Here's how the part is built. I have some questions about the finished solid (model axes, mm). Face numbers are marked on the shaded views. A direction names the side the tool comes from. Round coordinates to 2 decimals unless told otherwise and drop trailing zeros. Order: outer loops, then holes, each group sorted by start corner. A loop starts at its lowest first (then second) coordinate and runs counter-clockwise, first axis right, second up. Notation, with made-up numbers: (70, -39.75) -> (123, -39.75) arc R5 cw to (123, -31.75) -> close; hole circle Ø11 at (-14.75, 82). An arc over 180 degrees is marked (long way). Answer in a Markdown table with one row per item.
```python
from build123d import *

# Parameters (mm, degrees)
SKETCH_2_W          = 140
SKETCH_2_H          = 140
EXTRUDE_1_DEPTH     = 4
EXTRUDE_1_2_DEPTH   = 100
EXTRUDE_2_DEPTH     = 2
CUT_EXTRUDE_1_DEPTH = 105.5
SKETCH_6_R          = 6.5
CUT_EXTRUDE_2_DEPTH = 5
FILLET_1_R          = 10
CUT_EXTRUDE_3_REACH = 106


with BuildPart() as part:
    # Эскиз2 → Extrude 1 (new body)
    with BuildSketch(Plane(origin=(0, 0, 0), x_dir=(1, 0, 0), z_dir=(0, 1, 0))):
        Rectangle(SKETCH_2_W, SKETCH_2_H)
    extrude(amount=EXTRUDE_1_DEPTH)

    # Эскиз3 → Extrude 1 2 (add)
    with BuildSketch(Plane(origin=(0, 4, 0), x_dir=(1, 0, 0), z_dir=(0, 1, 0))):
        with BuildLine():
            Line((-30.5, -30), (-30.5, 29))
            ThreePointArc((-30.5, 29), (-30.207106781, 29.707106781), (-29.5, 30))
            Line((-29.5, 30), (29.5, 30))
            ThreePointArc((29.5, 30), (30.207106781, 29.707106781), (30.5, 29))
            Line((30.5, 29), (30.5, -30))
            Line((30.5, -30), (34.5, -30))
            Line((34.5, -30), (34.5, 29))
            ThreePointArc((34.5, 29), (33.035533906, 32.535533906), (29.5, 34))
            Line((29.5, 34), (-29.5, 34))
            ThreePointArc((-29.5, 34), (-33.035533906, 32.535533906), (-34.5, 29))
            Line((-34.5, 29), (-34.5, -30))
            Line((-34.5, -30), (-30.5, -30))
        make_face()
    extrude(amount=EXTRUDE_1_2_DEPTH)

    # Эскиз4 → Бобышка-Вытянуть2 (add, symmetric)
    with BuildSketch(Plane(origin=(0, 0, 0), x_dir=(0, 0, -1), z_dir=(1, 0, 0))):
        Polygon((34, 57.693575035), (65, 4), (34, 4), align=None)
    extrude(amount=EXTRUDE_2_DEPTH, both=True)

    # Эскиз5 → Вырез-Вытянуть1 (cut, through all)
    with BuildSketch(Plane(origin=(34.5, 0, 0), x_dir=(0, 0, -1), z_dir=(1, 0, 0))):
        with BuildLine():
            Line((-10, 92), (-10, 80))
            ThreePointArc((-10, 80), (-15, 75), (-20, 80))
            Line((-20, 80), (-20, 92))
            ThreePointArc((-20, 92), (-15, 97), (-10, 92))
        make_face()
        with BuildLine():
            Line((-10, 28), (-10, 16))
            ThreePointArc((-10, 16), (-15, 11), (-20, 16))
            Line((-20, 16), (-20, 28))
            ThreePointArc((-20, 28), (-15, 33), (-10, 28))
        make_face()
        with BuildLine():
            Line((10, 92), (10, 80))
            ThreePointArc((10, 80), (15, 75), (20, 80))
            Line((20, 80), (20, 92))
            ThreePointArc((20, 92), (15, 97), (10, 92))
        make_face()
        with BuildLine():
            Line((10, 28), (10, 16))
            ThreePointArc((10, 16), (15, 11), (20, 16))
            Line((20, 16), (20, 28))
            ThreePointArc((20, 28), (15, 33), (10, 28))
        make_face()
    extrude(amount=-CUT_EXTRUDE_1_DEPTH, mode=Mode.SUBTRACT)

    # Эскиз6 → Вырез-Вытянуть2 (cut, through all)
    with BuildSketch(Plane(origin=(0, 4, 0), x_dir=(1, 0, 0), z_dir=(0, 1, 0))):
        with Locations(Location((-55, 55, 0), (0, 0, 270))):  # turned: the seam where the file's is
            Circle(SKETCH_6_R)
        with Locations(Location((-55, -55, 0), (0, 0, 270))):  # turned: the seam where the file's is
            Circle(SKETCH_6_R)
        with Locations(Location((55, 55, 0), (0, 0, 270))):  # turned: the seam where the file's is
            Circle(SKETCH_6_R)
        with Locations(Location((55, -55, 0), (0, 0, 270))):  # turned: the seam where the file's is
            Circle(SKETCH_6_R)
    extrude(amount=-CUT_EXTRUDE_2_DEPTH, mode=Mode.SUBTRACT)

    # Скругление1
    fillet_1_edges = [part.edges().sort_by_distance(p)[0] for p in [
        (70, 2, 70),
        (-70, 2, 70),
        (-70, 2, -70),
        (70, 2, -70),
    ]]
    fillet(fillet_1_edges, radius=FILLET_1_R)

    # Эскиз8 → Вырез-Вытянуть3 (cut, up to next)
    with BuildSketch(Plane(origin=(0, 0, -34), x_dir=(-1, 0, 0), z_dir=(0, 0, -1)), mode=Mode.PRIVATE) as cut_extrude_3_sk1:
        with BuildLine():
            Line((-10, 92), (-10, 80))
            ThreePointArc((-10, 80), (-15, 75), (-20, 80))
            Line((-20, 80), (-20, 92))
            ThreePointArc((-20, 92), (-15, 97), (-10, 92))
        make_face()
    cut_extrude_3_tool1 = extrude(cut_extrude_3_sk1.sketch, amount=-CUT_EXTRUDE_3_REACH, mode=Mode.PRIVATE) & part.part
    add(cut_extrude_3_tool1.solids().sort_by_distance((15, 86, -34))[0], mode=Mode.SUBTRACT)
    # Эскиз8 → Вырез-Вытянуть3 (cut, up to next)
    with BuildSketch(Plane(origin=(0, 0, -34), x_dir=(-1, 0, 0), z_dir=(0, 0, -1)), mode=Mode.PRIVATE) as cut_extrude_3_sk2:
        with BuildLine():
            Line((-10, 28), (-10, 16))
            ThreePointArc((-10, 16), (-15, 11), (-20, 16))
            Line((-20, 16), (-20, 28))
            ThreePointArc((-20, 28), (-15, 33), (-10, 28))
        make_face()
    cut_extrude_3_tool2 = extrude(cut_extrude_3_sk2.sketch, amount=-CUT_EXTRUDE_3_REACH, mode=Mode.PRIVATE) & part.part
    add(cut_extrude_3_tool2.solids().sort_by_distance((15, 22, -34))[0], mode=Mode.SUBTRACT)
    # Эскиз8 → Вырез-Вытянуть3 (cut, up to next)
    with BuildSketch(Plane(origin=(0, 0, -34), x_dir=(-1, 0, 0), z_dir=(0, 0, -1)), mode=Mode.PRIVATE) as cut_extrude_3_sk3:
        with BuildLine():
            Line((10, 92), (10, 80))
            ThreePointArc((10, 80), (15, 75), (20, 80))
            Line((20, 80), (20, 92))
            ThreePointArc((20, 92), (15, 97), (10, 92))
        make_face()
    cut_extrude_3_tool3 = extrude(cut_extrude_3_sk3.sketch, amount=-CUT_EXTRUDE_3_REACH, mode=Mode.PRIVATE) & part.part
    add(cut_extrude_3_tool3.solids().sort_by_distance((-15, 86, -34))[0], mode=Mode.SUBTRACT)
    # Эскиз8 → Вырез-Вытянуть3 (cut, up to next)
    with BuildSketch(Plane(origin=(0, 0, -34), x_dir=(-1, 0, 0), z_dir=(0, 0, -1)), mode=Mode.PRIVATE) as cut_extrude_3_sk4:
        with BuildLine():
            Line((10, 28), (10, 16))
            ThreePointArc((10, 16), (15, 11), (20, 16))
            Line((20, 16), (20, 28))
            ThreePointArc((20, 28), (15, 33), (10, 28))
        make_face()
    cut_extrude_3_tool4 = extrude(cut_extrude_3_sk4.sketch, amount=-CUT_EXTRUDE_3_REACH, mode=Mode.PRIVATE) & part.part
    add(cut_extrude_3_tool4.solids().sort_by_distance((-15, 22, -34))[0], mode=Mode.SUBTRACT)


solid = part.part
```
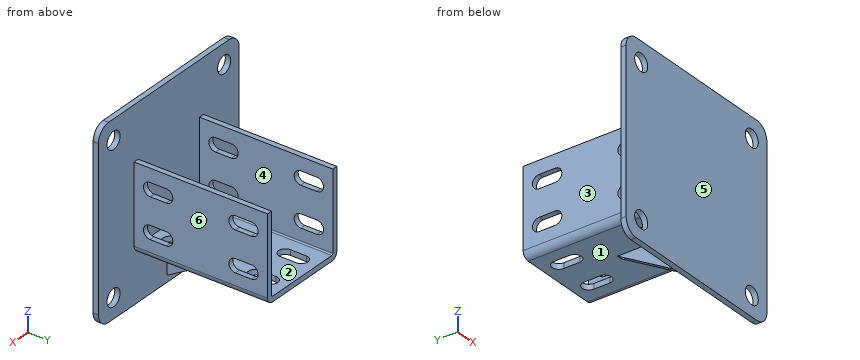
1. For the marked faces 1 and 2, which set-ups out of +Z, -Z, +X, -X, +Y, -Y let a thin tool reach every point of the face, with its end or its side?
Numbers:
| item | result |
|---|---|
| face 1 | -Z, +Y |
| face 2 | +Z, +Y |
2. For pin 1 Ø1.2 at (x, y) = (33, 88) entering from -Z; pin 2 Ø2 at (y, z) = (22, -32) entering from -X; pin 3 Ø3 at (x, z) = (-39, 53) entering from +Y, each with a flat end and sliding along its axis, tell me the tip position at first contact or that it passes through.
Numbers:
| item | result |
|---|---|
| pin 1 | stops at z = -33.07 |
| pin 2 | stops at x = -34.08 |
| pin 3 | stops at y = 4 |
3. We'd pull the mould along X, two halves only. Please class the marked faces 3, 4, 5 and 6: released by +X, released by -X, zero draft, split by the parting line, or undercut.
Numbers:
| item | result |
|---|---|
| face 3 | released by -X |
| face 4 | undercut |
| face 5 | zero draft |
| face 6 | released by +X |
4. Suppose I cut it at D-D on x = 15. Write out the boundary of the cut face in (y, z), then the cut area to 3 significant figures.
Numbers:
| item | result |
|---|---|
| outline | (0, -70) -> (4, -70) -> (4, -34) -> (11, -34) -> (11, -30) -> (4, -30) -> (4, 70) -> (0, 70) -> close; (33, -34) -> (75, -34) -> (75, -30) -> (33, -30) -> close; (97, -34) -> (104, -34) -> (104, -30) -> (97, -30) -> close |
| area | 784 mm2 |
5. Suppose I cut it at B-B on z = -15. Write out the boundary of the cut face in (x, y).
Numbers:
| item | result |
|---|---|
| outline | (-70, 0) -> (70, 0) -> (70, 4) -> (34.5, 4) -> (34.5, 11) -> (30.5, 11) -> (30.5, 4) -> (-30.5, 4) -> (-30.5, 11) -> (-34.5, 11) -> (-34.5, 4) -> (-70, 4) -> close; (-34.5, 33) -> (-30.5, 33) -> (-30.5, 75) -> (-34.5, 75) -> close; (-34.5, 97) -> (-30.5, 97) -> (-30.5, 104) -> (-34.5, 104) -> close; (30.5, 33) -> (34.5, 33) -> (34.5, 75) -> (30.5, 75) -> close; (30.5, 97) -> (34.5, 97) -> (34.5, 104) -> (30.5, 104) -> close |
6. Suppose I cut it at C-C on y = 61. Write out the boundary of the cut face in (x, z).
Numbers:
| item | result |
|---|---|
| outline | (-34.5, -29) arc R5 ccw to (-29.5, -34) -> (29.5, -34) arc R5 ccw to (34.5, -29) -> (34.5, 30) -> (30.5, 30) -> (30.5, -29) arc R1 cw to (29.5, -30) -> (-29.5, -30) arc R1 cw to (-30.5, -29) -> (-30.5, 30) -> (-34.5, 30) -> close |
7. Please list where these lines run through material, in increasing order: line 1 along X through (y, z) = (3.25, 55); line 2 along X through (y, z) = (87.5, -28); line 3 along Z through (x, y) = (33, 80).
Numbers:
| item | result |
|---|---|
| line 1 | x = -70 to -61.5, -48.5 to 48.5, 61.5 to 70 |
| line 2 | x = -34.5 to -30.5, 30.5 to 34.5 |
| line 3 | z = -32.57 to -20, -10 to 10, 20 to 30 |
8. Suppose I cut it at A-A on x = -55. Write out the boundary of the cut face in (y, z).
Numbers:
| item | result |
|---|---|
| outline | (0, -70) -> (4, -70) -> (4, -61.5) -> (0, -61.5) -> close; (0, -48.5) -> (4, -48.5) -> (4, 48.5) -> (0, 48.5) -> close; (0, 61.5) -> (4, 61.5) -> (4, 70) -> (0, 70) -> close |
